Model file for the job. Use its own axes, mm. Coordinates: 2 decimals unless noted, no trailing zeros. Write each loop counter-clockwise with the first axis right and the second up, starting at its lowest first coordinate (ties: lowest second). Pieces come first, ordered by that corner, then holes. Notation, with made-up numbers: M -24.5,77.5 L 26.5,77.5 A22 ccw 26.5,109.5 Z; hole C 30,-18.75 d2. An arc over 180 degrees is marked long. Put each result on its own line as item: value. Start each with the question number.
Q1. Drill centre lines: line 1 along X through (y, z) = (-29, 1.65); line 2 along Y through (x, z) = (74.5, 0.9); line 3 along X through (y, z) = (45, 0.85). Where is each one in solid material? Low to high.
Q2. Cut at C-C (z = 0.35). Give the number of separate pieces and of enclosed holes in the cut face, then the cut area to 3 significant figures.
Q3. Cut at D-D (x = -87.5). Write the cut outline in (y, z), then the cut area to 3 significant figures.
Q4. Cut at A-A (x = 90). Write the cut outline in (y, z), then the cut area to 3 significant figures.
Q5. Cut at B-B (y = 33). Write the cut outline in (x, z), then the cut area to 3 significant figures.
```python
from build123d import *

# Parameters (mm, degrees)
SKETCH_1_W            = 246
SKETCH_1_H            = 230
EXTRUDE_1_DEPTH       = 2
CUT_EXTRUDE_2_DEPTH   = 169.398337284
MIRROR_2_COPY_1_DEPTH = 169.398337284


with BuildPart() as part:
    # 草图1 → 凸台-拉伸1 (new body)
    with BuildSketch(Plane.XY):
        Rectangle(SKETCH_1_W, SKETCH_1_H)
    extrude(amount=EXTRUDE_1_DEPTH)

    # 草图2 → 切除-拉伸2 (cut, through all)
    with BuildSketch(Plane.XY.offset(2)):
        Polygon((-61.485344815, -28.880757709), (-97.255935728, -64.651348622), (-76.945987349, -64.651348622), (-61.5, -49.205361273), (-45.159781882, -65.545579391), (-25.813195161, -65.545579391), align=None)
        Polygon((-61.5, -64.03252581), (-97.255935728, -99.788461538), (-77.840218118, -99.788461538), (-61.5, -83.44824342), (-45.159781882, -99.788461538), (-25.744064272, -99.788461538), align=None)
    cut_extrude_2 = extrude(amount=-CUT_EXTRUDE_2_DEPTH, mode=Mode.SUBTRACT)

    # 镜向1: 切除-拉伸2 across plane
    add(cut_extrude_2.mirror(Plane.ZX), mode=Mode.SUBTRACT)

    # 镜向2: 切除-拉伸2 across plane
    add(cut_extrude_2.mirror(Plane(origin=(0, 0, 0), x_dir=(0, 0, 1), z_dir=(1, 0, 0))), mode=Mode.SUBTRACT)

    # 镜向2 copy 1 sketch → 镜向2 copy 1 (cut, through all)
    with BuildSketch(Plane(origin=(0, 0, 2), x_dir=(-1, 0, 0), z_dir=(0, 0, 1))):
        Polygon((-61.485344815, -28.880757709), (-97.255935728, -64.651348622), (-76.945987349, -64.651348622), (-61.5, -49.205361273), (-45.159781882, -65.545579391), (-25.813195161, -65.545579391), align=None)
        Polygon((-61.5, -64.03252581), (-97.255935728, -99.788461538), (-77.840218118, -99.788461538), (-61.5, -83.44824342), (-45.159781882, -99.788461538), (-25.744064272, -99.788461538), align=None)
    extrude(amount=-MIRROR_2_COPY_1_DEPTH, mode=Mode.SUBTRACT)


solid = part.part
```
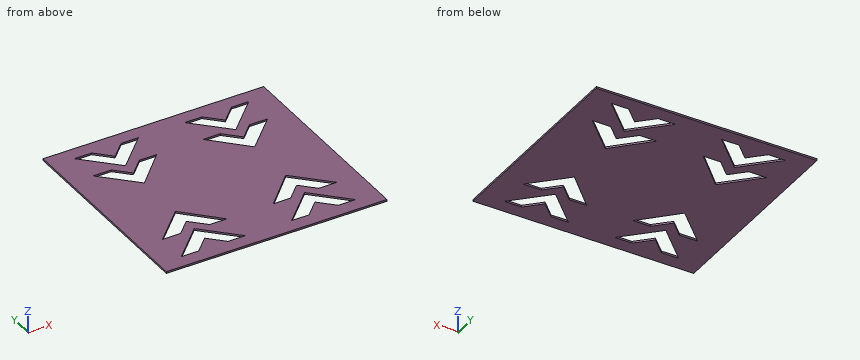
Computed values:
1. line 1: -123 to -61.6, -61.37 to 61.37, 61.6 to 123
1. line 2: -115 to -96.45, -77.03 to -62.21, -41.9 to 41.9, 62.21 to 77.03, 96.45 to 115
1. line 3: -123 to -77.6, -45.8 to 45.8, 77.6 to 123
2. separate pieces: 1
2. enclosed holes: 8
2. area: 48,400 mm2
3. outline: M -115,0 L -99.79,0 L -99.79,2 L -115,2 Z; M -90.03,0 L -64.65,0 L -64.65,2 L -90.03,2 Z; M -54.9,0 L 54.9,0 L 54.9,2 L -54.9,2 Z; M 64.65,0 L 90.03,0 L 90.03,2 L 64.65,2 Z; M 99.79,0 L 115,0 L 115,2 L 99.79,2 Z
3. area: 382 mm2
4. outline: M -115,0 L -99.79,0 L -99.79,2 L -115,2 Z; M -92.53,0 L -64.65,0 L -64.65,2 L -92.53,2 Z; M -57.4,0 L 57.4,0 L 57.4,2 L -57.4,2 Z; M 64.65,0 L 92.53,0 L 92.53,2 L 64.65,2 Z; M 99.79,0 L 115,0 L 115,2 L 99.79,2 Z
4. area: 402 mm2
5. outline: M -123,0 L -65.6,0 L -65.6,2 L -123,2 Z; M -57.48,0 L 57.48,0 L 57.48,2 L -57.48,2 Z; M 65.6,0 L 123,0 L 123,2 L 65.6,2 Z
5. area: 459 mm2
